For this review, use the dimensioned drawing (mm, ordinates from the lowest corner) and the shaded views. Round coordinates to 2 decimals unless told otherwise and drop trailing zeros. Order: outer loops, then holes, each group sorted by start corner. A loop starts at its lowest first (then second) coordinate and runs counter-clockwise, first axis right, second up. Notation, with made-up numbers: M 65,-24.5 L 107,-24.5 A25 cw 107,10.5 Z; hole C 57.5,2.5 d7. An arc over 180 degrees is marked long. Use a Markdown table: item, result. Add a question column.
1. The part is to be moulded in two halves that separate along Z. For the marked faces 1 and 2, say which applies: +Z half, -Z half, draft (parallel to the pull), parting line (faces both ways), or undercut.
2. Consider section B-B on y = 15. State the section outline as (x, z) points, then the cut area to 3 significant figures.
3. Insertion check: P1, Ø1.9, axis at y = 15.5, z = 3, coming from the -X side; P2, Ø1.9, axis at y = 36.5, z = 2, coming from the +X side; P3, Ø3, axis at x = 150, z = 4, coming from the +Y side. Each pin has a flat end and moves straight along its axis. Give the tip position at first contact, or say it passes through.
4. To check wall thickness, follow probe 1 along X at (y, z) = (48.5, 2); probe 2 along X at (y, z) = (32.5, 5.75); probe 3 along Y at (x, z) = (154.5, 3). State the ranges of each line that lie inside material, in increasing order.
5. Consider section A-A on z = 5.25. State the section outline as (x, y) points, then the cut area to 3 significant figures.
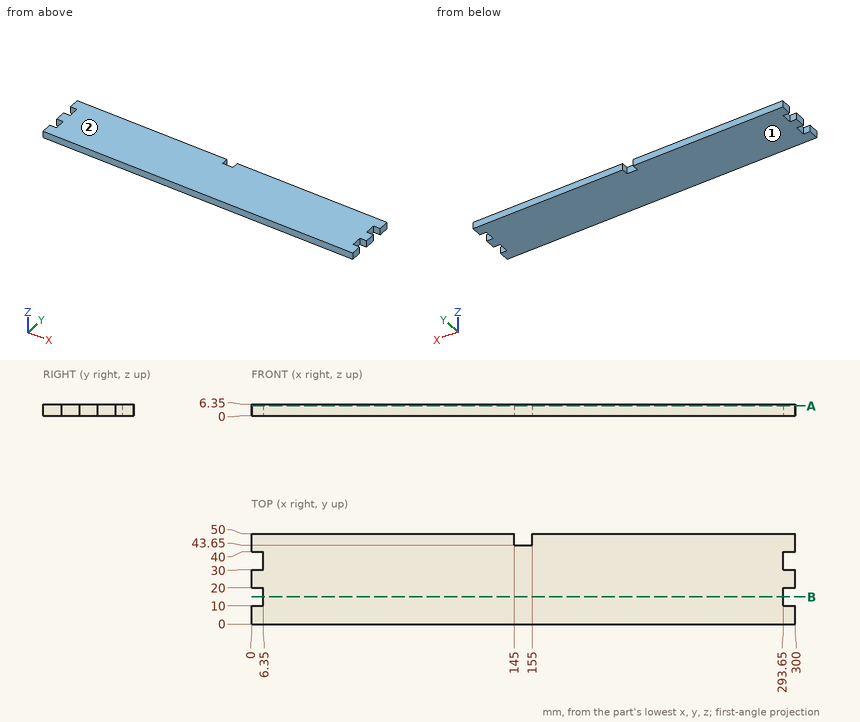
Answer block:
| question | item | result |
|---|---|---|
| 1 | face 1 | -Z half |
| 1 | face 2 | +Z half |
| 2 | outline | M 6.35,0 L 293.65,0 L 293.65,6.35 L 6.35,6.35 Z |
| 2 | area | 1,820 mm^2 |
| 3 | P1 | x = 6.35 |
| 3 | P2 | x = 293.65 |
| 3 | P3 | y = 43.65 |
| 4 | probe 1 | 0 to 145, 155 to 300 |
| 4 | probe 2 | 6.35 to 293.65 |
| 4 | probe 3 | 0 to 43.65 |
| 5 | outline | M 0,0 L 300,0 L 300,10 L 293.65,10 L 293.65,20 L 300,20 L 300,30 L 293.65,30 L 293.65,40 L 300,40 L 300,50 L 155,50 L 155,43.65 L 145,43.65 L 145,50 L 0,50 L 0,40 L 6.35,40 L 6.35,30 L 0,30 L 0,20 L 6.35,20 L 6.35,10 L 0,10 Z |
| 5 | area | 14,700 mm^2 |
